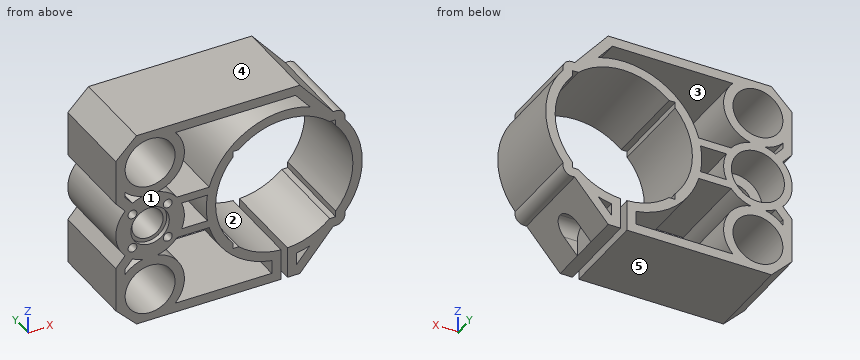
from build123d import *

# Parameters (mm, degrees)
SKETCH1_R           = 8
SKETCH1_R_2         = 8.5
BOSS_EXTRUDE1_DEPTH = 28
BOSS_EXTRUDE3_DEPTH = 12
CUT_EXTRUDE1_DEPTH  = 14.407172
SKETCH7_R           = 8.5
BOSS_EXTRUDE4_DEPTH = 15
SKETCH7_3_R         = 5
CUT_EXTRUDE2_DEPTH  = 15
SKETCH7_4_R         = 6.165
CUT_EXTRUDE3_DEPTH  = 1.5
SKETCH7_5_R         = 1.425
CUT_EXTRUDE4_DEPTH  = 8


with BuildPart() as part:
    # Sketch1 → Boss-Extrude1 (new body)
    with BuildSketch(Plane(origin=(0, 0, 0), x_dir=(1, 0, 0), z_dir=(0, 1, 0))):
        with BuildLine():
            ThreePointArc((-50.982546594, 7.568285795), (-54, 0), (-50.982546594, -7.568285795))
            Line((-50.982546594, -7.568285795), (-54, -11))
            Line((-54, -11), (-54, -25.34082208))
            Line((-54, -25.34082208), (-47.34082208, -32))
            Line((-47.34082208, -32), (5, -32))
            Line((5, -32), (15.759494281, -19.407172386))
            ThreePointArc((15.759494281, -19.407172386), (18.621320344, -18.621320344), (19.407172386, -15.759494281))
            ThreePointArc((19.407172386, -15.759494281), (25, 0), (19.407172386, 15.759494281))
            ThreePointArc((19.407172386, 15.759494281), (18.621320344, 18.621320344), (15.759494281, 19.407172386))
            Line((15.759494281, 19.407172386), (5, 32))
            Line((5, 32), (1, 32))
            Line((1, 32), (1, 21.977260976))
            ThreePointArc((1, 21.977260976), (8.243992543, 20.396974946), (14.551632211, 16.5))
            Line((14.551632211, 16.5), (16.5, 16.5))
            Line((16.5, 16.5), (16.5, 14.551632211))
            ThreePointArc((16.5, 14.551632211), (22, 0), (16.5, -14.551632211))
            Line((16.5, -14.551632211), (16.5, -16.5))
            Line((16.5, -16.5), (14.551632211, -16.5))
            ThreePointArc((14.551632211, -16.5), (0, -22), (-14.551632211, -16.5))
            Line((-14.551632211, -16.5), (-16.5, -16.5))
            Line((-16.5, -16.5), (-16.5, -14.551632211))
            ThreePointArc((-16.5, -14.551632211), (-22, 0), (-16.5, 14.551632211))
            Line((-16.5, 14.551632211), (-16.5, 16.5))
            Line((-16.5, 16.5), (-14.551632211, 16.5))
            ThreePointArc((-14.551632211, 16.5), (-8.243992543, 20.396974946), (-1, 21.977260976))
            Line((-1, 21.977260976), (-1, 32))
            Line((-1, 32), (-47.34082208, 32))
            Line((-47.34082208, 32), (-54, 25.34082208))
            Line((-54, 25.34082208), (-54, 11))
            Line((-54, 11), (-50.982546594, 7.568285795))
        make_face()
        with BuildLine():
            ThreePointArc((-48.638105805, -9.445197877), (-47.038026147, -10.232025451), (-45.331844763, -10.75))
            ThreePointArc((-45.331844763, -10.75), (-48.408051309, -11.921222362), (-51, -13.950165565))
            Line((-51, -13.950165565), (-51, -12.131352314))
            Line((-51, -12.131352314), (-48.638105805, -9.445197877))
        make_face(mode=Mode.SUBTRACT)
        with Locations((-43, -21.5)):
            Circle(SKETCH1_R, mode=Mode.SUBTRACT)
        with BuildLine():
            ThreePointArc((-34.95326153, -29), (-32.502649264, -18.212808567), (-40.668155237, -10.75))
            ThreePointArc((-40.668155237, -10.75), (-37.204464997, -9.349426401), (-34.409357086, -6.870287791))
            Line((-34.409357086, -6.870287791), (-24.037452978, -6.870287791))
            ThreePointArc((-24.037452978, -6.870287791), (-11.513133706, -22.191163833), (8.224630177, -23.60837687))
            Line((8.224630177, -23.60837687), (3.617949295, -29))
            Line((3.617949295, -29), (-34.95326153, -29))
        make_face(mode=Mode.SUBTRACT)
        with Locations((-43, 0)):
            Circle(SKETCH1_R_2, mode=Mode.SUBTRACT)
        with BuildLine():
            ThreePointArc((-45.331844763, 10.75), (-47.038026147, 10.232025451), (-48.638105805, 9.445197877))
            Line((-48.638105805, 9.445197877), (-51, 12.131352314))
            Line((-51, 12.131352314), (-51, 13.950165565))
            ThreePointArc((-51, 13.950165565), (-48.408051309, 11.921222362), (-45.331844763, 10.75))
        make_face(mode=Mode.SUBTRACT)
        with BuildLine():
            ThreePointArc((-32.905418056, -4.370287791), (-32, 0), (-32.905418056, 4.370287791))
            Line((-32.905418056, 4.370287791), (-24.615047931, 4.370287791))
            ThreePointArc((-24.615047931, 4.370287791), (-25, 0), (-24.615047931, -4.370287791))
            Line((-24.615047931, -4.370287791), (-32.905418056, -4.370287791))
        make_face(mode=Mode.SUBTRACT)
        with Locations((-43, 21.5)):
            Circle(SKETCH1_R, mode=Mode.SUBTRACT)
        with BuildLine():
            ThreePointArc((-34.409357086, 6.870287791), (-37.204464997, 9.349426401), (-40.668155237, 10.75))
            ThreePointArc((-40.668155237, 10.75), (-32.502649264, 18.212808567), (-34.95326153, 29))
            Line((-34.95326153, 29), (-4, 29))
            Line((-4, 29), (-4, 24.677925359))
            ThreePointArc((-4, 24.677925359), (-16.607308069, 18.68682206), (-24.037452978, 6.870287791))
            Line((-24.037452978, 6.870287791), (-34.409357086, 6.870287791))
        make_face(mode=Mode.SUBTRACT)
        with BuildLine():
            ThreePointArc((8.223751321, 23.608683026), (6.135213434, 24.235493725), (4, 24.677925359))
            Line((4, 24.677925359), (4, 28.552128404))
            Line((4, 28.552128404), (8.223751321, 23.608683026))
        make_face(mode=Mode.SUBTRACT)
    extrude(amount=BOSS_EXTRUDE1_DEPTH)

    # Sketch6 → Boss-Extrude3 (add)
    with BuildSketch(Plane(origin=(0, 20, 0), x_dir=(0, 0, -1), z_dir=(0, -1, 0))):
        Polygon((30.717367885, 3.963704263), (22.785433959, 3.963704263), (22.785433959, 10.604126234), align=None)
    extrude(amount=BOSS_EXTRUDE3_DEPTH)

    # Sketch3 → Cut-Extrude1 (cut)
    with BuildSketch(Plane.ZY.offset(-19.407172386)):
        with BuildLine():
            ThreePointArc((-23, 14), (-24.171572875, 16.828427125), (-27, 18))
            Line((-27, 18), (-27, 10))
            ThreePointArc((-27, 10), (-24.171572875, 11.171572875), (-23, 14))
        make_face()
        with BuildLine():
            Line((-27, 10), (-27, 18))
            ThreePointArc((-27, 18), (-31, 14), (-27, 10))
        make_face()
        with BuildLine():
            Line((-27, 18), (-32, 18))
            Line((-32, 18), (-32, 10))
            Line((-32, 10), (-27, 10))
            ThreePointArc((-27, 10), (-31, 14), (-27, 18))
        make_face()
    extrude(amount=CUT_EXTRUDE1_DEPTH, mode=Mode.SUBTRACT)

    # Sketch7 → Boss-Extrude4 (add)
    with BuildSketch(Plane.XZ):
        with Locations((-43, 0)):
            Circle(SKETCH7_R)
    extrude(amount=-BOSS_EXTRUDE4_DEPTH)

    # Sketch7<3> → Cut-Extrude2 (cut)
    with BuildSketch(Plane.XZ):
        with Locations((-43, 0)):
            Circle(SKETCH7_3_R)
    extrude(amount=-CUT_EXTRUDE2_DEPTH, mode=Mode.SUBTRACT)

    # Sketch7<4> → Cut-Extrude3 (cut)
    with BuildSketch(Plane.XZ):
        with Locations((-43, 0)):
            Circle(SKETCH7_4_R)
    extrude(amount=-CUT_EXTRUDE3_DEPTH, mode=Mode.SUBTRACT)

    # Sketch7<5> → Cut-Extrude4 (cut)
    with BuildSketch(Plane.XZ):
        with Locations((-48.64603005, -5.667657777)):
            Circle(SKETCH7_5_R)
        with Locations((-48.656854249, 5.656854249)):
            Circle(SKETCH7_5_R)
        with Locations((-37.332342223, 5.667678449)):
            Circle(SKETCH7_5_R)
        with Locations((-37.321518023, -5.656833577)):
            Circle(SKETCH7_5_R)
    extrude(amount=-CUT_EXTRUDE4_DEPTH, mode=Mode.SUBTRACT)


solid = part.part
For this review, take the finished solid that the model builds, in its own axes (mm). Face numbers are marked on the shaded views. A direction names the side the tool comes from. Round coordinates to 2 decimals unless told otherwise and drop trailing zeros. Write each loop counter-clockwise with the first axis right and the second up, starting at its lowest first coordinate (ties: lowest second). Pieces come first, ordered by that corner, then holes. Notation, with made-up numbers: M 71.5,56.5 L 80.5,56.5 A35 cw 80.5,89.5 Z; hole C 24.5,56.5 d7. An arc over 180 degrees is marked long. Write item = value, one per line. Start each with the question number.
(1) We need section D-D (x = 18.5). Give the boundary of the cut face in (y, z).
(2) Clearance check with flat-ended pins moving along their axes: pin 1 Ø0.5 at (y, z) = (19, -13) entering from +X; pin 2 Ø1.3 at (y, z) = (7, -27.5) entering from -X; pin 3 Ø10 at (x, y) = (11, 23) entering from -Z; pin 4 Ø3 at (x, z) = (10.5, 16.5) entering from -Y. State where each tip first meets the part, or that it passes through.
(3) We need section C-C (y = 23.25). Give the number of separate pieces and of enclosed holes in the cut face, then the cut area to 3 significant figures.
(4) We need section A-A (z = 0). Give the boundary of the cut face in (x, y) (3 decimals), then the cut area to 3 significant figures.
(5) We need section B-B (x = -43). Give the boundary of the cut face in (y, z) (3 decimals), then the cut area to 3 significant figures.
(6) The part is to be moulded in two halves that separate along Z. For the marked faces 3, 4 and 5, say which applies: +Z half, -Z half, draft (parallel to the pull), parting line (faces both ways), or undercut.
(7) For the marked faces 1 and 2, list the 3-axis set-ups (+Z, -Z, +X, -X, +Y, -Y) from which the entire face can be reached by the end or side of a thin tool; tool diameter is ignored.
(8) For line 1 along Z through (x, y) = (-43, 19); line 2 along Z through (x, y) = (-43, 7); line 3 along X through (y, z) = (23.25, -1), list the stretches that pass through material, from the lowest coordinate up.
Results found:
q1.outline = M 0,-18.74 L 28,-18.74 L 28,-11.91 L 0,-11.91 Z; M 0,11.91 L 28,11.91 L 28,18.74 L 0,18.74 Z
q2.pin_1 = 21.5
q2.pin_2 = -52.49
q2.pin_3 = -30.83
q2.pin_4 = through
q3.separate_pieces = 1
q3.enclosed_holes = 9
q3.area = 1,370 mm²
q4.outline = M -54,0 L -49.165,0 L -49.165,1.5 L -48,1.5 L -48,15 L -51.5,15 L -51.5,28 L -54,28 Z; M -38,1.5 L -36.835,1.5 L -36.835,0 L -32,0 L -32,28 L -34.5,28 L -34.5,15 L -38,15 Z; M -25,0 L -22,0 L -22,28 L -25,28 Z; M 22,0 L 25,0 L 25,28 L 22,28 Z
q4.area = 410 mm²
q5.outline = M 0,-32 L 28,-32 L 28,-29.5 L 0,-29.5 Z; M 0,-13.5 L 28,-13.5 L 28,-8.5 L 15,-8.5 L 15,-5 L 1.5,-5 L 1.5,-6.165 L 0,-6.165 Z; M 0,6.165 L 1.5,6.165 L 1.5,5 L 15,5 L 15,8.5 L 28,8.5 L 28,13.5 L 0,13.5 Z; M 0,29.5 L 28,29.5 L 28,32 L 0,32 Z
q5.area = 522 mm²
q6.face_3 = undercut
q6.face_4 = +Z half
q6.face_5 = -Z half
q7.face_1 = +Z, -Z, +X, -X, -Y
q7.face_2 = +Y, -Y
q8.line_1 = -32 to -29.5, -13.5 to -8.5, 8.5 to 13.5, 29.5 to 32
q8.line_2 = -32 to -29.5, -13.5 to -5, 5 to 13.5, 29.5 to 32
q8.line_3 = -53.95 to -51.44, -34.56 to -32.05, -24.98 to -21.98, 21.98 to 24.98
